```python
from build123d import *

# Parameters (mm, degrees)
GEARFACEPROFILE_R        = 15
GEARFACEEXTRUDE_DEPTH    = 15
CENTERSLOT_DEPTH         = 26.980762114
GEARCONNECTORS_OUTLINE_R = 3.5
GEARCONNECTORS_DEPTH     = 3.8


# Read off the part's stored shape, not the designer's step: GearConnectors
with BuildPart() as part:
    # GearFaceProfile → GearFaceExtrude (new body)
    with BuildSketch(Plane.XY):
        Circle(GEARFACEPROFILE_R)
    extrude(amount=GEARFACEEXTRUDE_DEPTH)

    # Sketch1 → CenterSlot (cut, through all)
    with BuildSketch(Plane.XY.offset(15)):
        with BuildLine():
            Line((-1.335, 6.504411964), (-1.335, 4.704411964))
            Line((-1.335, 4.704411964), (1.335, 4.704411964))
            Line((1.335, 4.704411964), (1.335, 6.504411964))
            ThreePointArc((1.335, 6.504411964), (0, -6.64), (-1.335, 6.504411964))
        make_face()
    extrude(amount=-CENTERSLOT_DEPTH, mode=Mode.SUBTRACT)

    # GearConnectors outline → GearConnectors (add)
    with BuildSketch(Plane(origin=(0, 0, 0), x_dir=(-1, 0, 0), z_dir=(0, 0, -1))):
        with BuildLine():
            ThreePointArc((5.310262334, -3.986315836), (11.691342952, -6.749999998), (6.107381948, -2.605664164))
            ThreePointArc((6.107381948, -2.605664164), (5.750408681, -3.32), (5.310262334, -3.986315836))
        make_face()
        with BuildLine():
            ThreePointArc((-6.107381948, -2.605664164), (-11.691342952, -6.749999998), (-5.310262334, -3.986315836))
            ThreePointArc((-5.310262334, -3.986315836), (-5.750408681, -3.32), (-6.107381948, -2.605664164))
        make_face()
        with Locations((0, 10)):
            Circle(GEARCONNECTORS_OUTLINE_R)
    extrude(amount=GEARCONNECTORS_DEPTH)


solid = part.part
```
Model file for the job. Use its own axes, mm. A direction names the side the tool comes from. Coordinates: 2 decimals unless noted, no trailing zeros. Order: outer loops, then holes, each group sorted by start corner. A loop starts at its lowest first (then second) coordinate and runs counter-clockwise, first axis right, second up. Notation, with made-up numbers: (29.25, 28) -> (39.25, 28) arc R18 cw to (39.25, 49) -> close; hole circle Ø6 at (29, -18). An arc over 180 degrees is marked (long way). Return JSON: item names as keys, results as strings.
Item 1: Slice it at A-A (x = 0). Write the cut outline in (y, z), then the cut area to 3 significant figures.
Model answer:
{"outline": "(-15, 0) -> (-6.64, 0) -> (-6.64, 15) -> (-15, 15) -> close; (4.7, 0) -> (6.5, 0) -> (6.5, -3.8) -> (13.5, -3.8) -> (13.5, 0) -> (15, 0) -> (15, 15) -> (4.7, 15) -> close", "area": "306 mm²"}
Item 2: Slice it at B-B (y = 0). Write the cut outline in (x, z), then the cut area to 3 significant figures.
Model answer:
{"outline": "(-15, 0) -> (-6.64, 0) -> (-6.64, 15) -> (-15, 15) -> close; (6.64, 0) -> (15, 0) -> (15, 15) -> (6.64, 15) -> close", "area": "251 mm²"}
Item 3: Pin check, flat tips, straight feed: P1, Ø4, axis at x = 7.5, y = 8, coming from the -Z side; P2, Ø0.5, axis at y = 6, z = 6.5, coming from the +X side; P3, Ø4, axis at x = 2.5, z = 6.5, coming from the -Y side. Stop position of each tip, or through.
Model answer:
{"P1": "stops at z = 0", "P2": "stops at x = 13.85", "P3": "stops at y = -14.99"}
Item 4: Wall check: line 1 along Z through (x, y) = (9.75, 5); line 2 along X through (y, z) = (3.25, 9.75); line 3 along X through (y, z) = (2.25, 0.75). Give the ranges that are in metal, low to high. Write a range as from..to.
Model answer:
{"line 1": "z = 0..15", "line 2": "x = -14.64..-5.79, 5.79..14.64", "line 3": "x = -14.83..-6.25, 6.25..14.83"}
Item 5: Slice it at C-C (z = 8.5). Write the cut outline in (x, y) (3 decimals).
Model answer:
{"outline": "circle Ø30 at (0, 0); hole (-1.335, 4.704) -> (-1.335, 6.504) arc R6.64 ccw (long way) to (1.335, 6.504) -> (1.335, 4.704) -> close"}
Item 6: 3-axis set-ups, long thin cutter, end or side, ignore diameter. For faces 4 (the face through (-9, -5, -3.8)), 5 (the face through (-11.6, -6.9, -1.9)), 6 (the face through (0, 4.704, 8)): which of +Z, -Z, +X, -X, +Y, -Y reach the whole face in a straight line?
Model answer:
{"face 4": "-Z, +X, -X, +Y, -Y", "face 5": "-Z", "face 6": "+Z, -Z"}
Item 7: Mould opens along Y. For faces 1 (the face through (0.759, 6.583, -1.873)), 2 (the face through (-1.335, 6, 8)), 3 (the face through (3.1, -6.5, 15)) say: pulls with the +Y half, pulls with the -Y half, needs draft (parallel to the pull), parting line crosses it, or undercut.
Model answer:
{"face 1": "parting line crosses it", "face 2": "undercut", "face 3": "needs draft"}
Item 8: Slice it at D-D (y = 10). Write the cut outline in (x, z), then the cut area to 3 significant figures.
Model answer:
{"outline": "(-11.18, 0) -> (-3.5, 0) -> (-3.5, -3.8) -> (3.5, -3.8) -> (3.5, 0) -> (11.18, 0) -> (11.18, 15) -> (-11.18, 15) -> close", "area": "362 mm²"}
